Part model, mm, in its own coordinate system. A direction names the side the tool comes from. Round coordinates to 2 decimals unless told otherwise and drop trailing zeros. Order: outer loops, then holes, each group sorted by start corner. A loop starts at its lowest first (then second) coordinate and runs counter-clockwise, first axis right, second up. Notation, with made-up numbers: (17, -19) -> (51, -19) arc R28 ccw to (51, 11) -> close; hole circle Ø9 at (19, -33.5). An arc over 180 degrees is marked (long way). Use CSV: the item, a comma, the result in double quotes.
```python
from build123d import *


with BuildPart() as part:
    # Esboço1 → Revolução1 (revolve)
    with BuildSketch(Plane.XY, mode=Mode.PRIVATE) as revolu_o1_sk:
        with BuildLine():
            Line((29.7, 13.740559465), (35.5, 13.740559465))
            Line((35.5, 13.740559465), (35.5, 1.740559465))
            Line((35.5, 1.740559465), (37, 1.740559465))
            Line((37, 1.740559465), (37, -20.259440535))
            Line((37, -20.259440535), (58.5, -20.259440535))
            Line((58.5, -20.259440535), (58.5, -30.259440535))
            Line((58.5, -30.259440535), (29.5, -30.259440535))
            Line((29.5, -30.259440535), (29.5, -35.259440535))
            Line((29.5, -35.259440535), (29, -35.259440535))
            Line((29, -35.259440535), (29, -47.259440535))
            Line((29, -47.259440535), (26, -47.259440535))
            Line((26, -47.259440535), (26, -36.259440535))
            Line((26, -36.259440535), (25.8, -36.259440535))
            Line((25.8, -36.259440535), (25.8, -25.459440535))
            ThreePointArc((25.8, -25.459440535), (27.05755123, -23.383232322), (27.189114949, -20.959440535))
            Line((27.189114949, -20.959440535), (27.189114949, -18.209440535))
            ThreePointArc((27.189114949, -18.209440535), (28.290718341, -13.494165971), (25.4, -9.609440535))
            Line((25.4, -9.609440535), (25.4, -1.859440535))
            ThreePointArc((25.4, -1.859440535), (28.290718341, 2.025284902), (27.189114949, 6.740559465))
            Line((27.189114949, 6.740559465), (27.189114949, 9.490559465))
            Line((27.189114949, 9.490559465), (29.7, 13.740559465))
        make_face()
    revolve(revolu_o1_sk.sketch.rotate(Axis((0, -64.843062606, 0), (0, 1, 0)), 90), axis=Axis((0, -64.843062606, 0), (0, 1, 0)))


solid = part.part
```
(1) Cut at A-A, the plane x = 32. Give the cut face in (y, z), then the cut area to 3 significant figures.
Reply:
outline,"(-30.26, -48.97) -> (-20.26, -48.97) -> (-20.26, -18.57) -> (1.74, -18.57) -> (1.74, -15.37) -> (13.74, -15.37) -> (13.74, 15.37) -> (1.74, 15.37) -> (1.74, 18.57) -> (-20.26, 18.57) -> (-20.26, 48.97) -> (-30.26, 48.97) -> close"
area,"2,170 mm2"
(2) Which spindle directions (+Z, -Z, +X, -X, +Y, -Y) get a long thin tool onto all of the face, cutting with end or side? Do faces 5 (the face through (29, 13.741, -8)), 6 (the face through (-14, -30.259, 27)), 7 (the face through (16.54, -19.57, 21.58)), 8 (the face through (34.656, 7.657, 7.696)). Say none if no direction does.
Reply:
face 5,"+Z, -Z, +X, -X, +Y"
face 6,"-Y"
face 7,"none"
face 8,"+Y"
(3) Pull direction Z, two halves, no side cores. Call faces 1 (the face through (16.54, 8.13, 21.58)), 2 (the face through (25.73, -41.34, -13.38)), 3 (the face through (-14, 1.741, -33)), 4 (the face through (15.821, -41.682, 20.633)): released by +Z, released by -Z, zero draft, split by the parting line, or undercut.
Reply:
face 1,"undercut"
face 2,"split by the parting line"
face 3,"zero draft"
face 4,"undercut"
(4) Drop flat-ended pins along their axis: P1, Ø12, axis at x = 36, z = 42, coming from the +Y side; P2, Ø10, axis at y = -10.5, z = -34, coming from the +X side; P3, Ø3, axis at y = -25.5, z = -24, coming from the +X side. Give the stop position or say it passes through.
Reply:
P1,"y = -20.26"
P2,"x = 22.98"
P3,"x = 54"
(5) Cut at B-B, the plane z = 51. Give the cut face in (x, y).
Reply:
outline,"(-28.66, -30.26) -> (28.66, -30.26) -> (28.66, -20.26) -> (-28.66, -20.26) -> close"
(6) Cut at C-C, the plane x = 46. Give the cut face in (y, z), then the cut area to 3 significant figures.
Reply:
outline,"(-30.26, -36.14) -> (-20.26, -36.14) -> (-20.26, 36.14) -> (-30.26, 36.14) -> close"
area,"723 mm2"
(7) Probe probe 1 along X at (y, z) = (7.9, 0); probe 2 along X at (y, z) = (-32.25, 0); probe 3 along Y at (x, z) = (37.5, 36.5). List the from-to ranges inside material, lowest first. Write a range as [from, to].
Reply:
probe 1,"[-35.5, -27.19], [27.19, 35.5]"
probe 2,"[-29.5, -25.8], [25.8, 29.5]"
probe 3,"[-30.26, -20.26]"
